Build history of the part. All positions in model axes, mm. A direction names the side the tool comes from. Give positions to 0.01 mm unless a question says otherwise; leave off trailing zeros. Order: outer loops, then holes, each group sorted by start corner. A loop starts at its lowest first (then second) coordinate and runs counter-clockwise, first axis right, second up. Notation, with made-up numbers: M 18.25,-23.5 L 48.25,-23.5 A22 cw 48.25,-6.5 Z; hole C 31.5,34 d11. An arc over 180 degrees is marked long. One line per item, written item: value.
from build123d import *

# Parameters (mm, degrees)
SKETCH1_R                                           = 14
BOSS_EXTRUDE1_DEPTH                                 = 37
SKETCH2_W                                           = 37
SKETCH2_H                                           = 37
BOSS_EXTRUDE2_DEPTH                                 = 6
CUT_EXTRUDE1_DEPTH                                  = 46.315560241
CBORE_FOR_M4_HEX_SOCKET_HEAD_CAP_SCREW1_D           = 4.5
CBORE_FOR_M4_HEX_SOCKET_HEAD_CAP_SCREW1_DEPTH       = 22
CBORE_FOR_M4_HEX_SOCKET_HEAD_CAP_SCREW1_CBORE_D     = 8
CBORE_FOR_M4_HEX_SOCKET_HEAD_CAP_SCREW1_CBORE_DEPTH = 4.4
CBORE_FOR_M4_HEX_SOCKET_HEAD_CAP_SCREW1_TIP         = 1.351936393
SKETCH8_R                                           = 8
CUT_EXTRUDE2_DEPTH                                  = 46.315560241
CHAMFER1_SIZE                                       = 1


with BuildPart() as part:
    # Sketch1 → Boss-Extrude1 (new body)
    with BuildSketch(Plane.XY):
        Circle(SKETCH1_R)
    extrude(amount=BOSS_EXTRUDE1_DEPTH)

    # Sketch2 → Boss-Extrude2 (add)
    with BuildSketch(Plane.XY.offset(37)):
        Rectangle(SKETCH2_W, SKETCH2_H)
    extrude(amount=-BOSS_EXTRUDE2_DEPTH)

    # Sketch4 → Cut-Extrude1 (cut, through all)
    with BuildSketch(Plane.XY.offset(37)):
        Polygon((-18.5, 18.5), (-18.5, 15.441125497), (-15.441125497, 18.5), align=None)
        Polygon((15.441125497, 18.5), (18.5, 18.5), (18.5, 15.441125497), align=None)
        Polygon((18.5, -18.5), (18.5, -15.441125497), (15.441125497, -18.5), align=None)
        Polygon((-15.441125497, -18.5), (-18.5, -18.5), (-18.5, -15.441125497), align=None)
    extrude(amount=-CUT_EXTRUDE1_DEPTH, mode=Mode.SUBTRACT)

    # CBORE for M4 Hex Socket Head Cap Screw1
    with Locations(Plane.XY.offset(37)):
        with Locations((-13.435028843, 13.435028843), (13.435028843, 13.435028843), (13.435028843, -13.435028843), (-13.435028843, -13.435028843)):
            CounterBoreHole(CBORE_FOR_M4_HEX_SOCKET_HEAD_CAP_SCREW1_D / 2, CBORE_FOR_M4_HEX_SOCKET_HEAD_CAP_SCREW1_CBORE_D / 2, CBORE_FOR_M4_HEX_SOCKET_HEAD_CAP_SCREW1_CBORE_DEPTH, depth=CBORE_FOR_M4_HEX_SOCKET_HEAD_CAP_SCREW1_DEPTH)
            with Locations((0, 0, -(CBORE_FOR_M4_HEX_SOCKET_HEAD_CAP_SCREW1_DEPTH + CBORE_FOR_M4_HEX_SOCKET_HEAD_CAP_SCREW1_TIP / 2))):  # 118° drill point
                Cone(0, CBORE_FOR_M4_HEX_SOCKET_HEAD_CAP_SCREW1_D / 2, CBORE_FOR_M4_HEX_SOCKET_HEAD_CAP_SCREW1_TIP, mode=Mode.SUBTRACT)

    # Sketch8 → Cut-Extrude2 (cut, through all)
    with BuildSketch(Plane.XY.offset(37)):
        Circle(SKETCH8_R)
    extrude(amount=-CUT_EXTRUDE2_DEPTH, mode=Mode.SUBTRACT)

    # Chamfer1
    chamfer1_edges = [part.edges().sort_by_distance(p)[0] for p in [
        (-8, 0, 37),
        (-14, 0, 0),
    ]]
    chamfer(chamfer1_edges, length=CHAMFER1_SIZE)


solid = part.part
1) Saw through at A-A, the plane y = 0. Write the cut outline in (x, z).
Check values:
outline: M -18.5,31 L -14,31 L -14,1 L -13,0 L -8,0 L -8,36 L -9,37 L -18.5,37 Z; M 8,0 L 13,0 L 14,1 L 14,31 L 18.5,31 L 18.5,37 L 9,37 L 8,36 Z
2) Mould opens along X. For faces 1 (the face through (6, 6, 0)), 2 (the face through (-16.99, -16.95, 34.04)), 3 (the face through (-9.62, -12.23, 34.83)) say: released by +X, released by -X, zero draft, split by the parting line, or undercut.
Check values:
face 1: zero draft
face 2: released by -X
face 3: undercut
3) Pin check, flat tips, straight feed: pin 1 (9 mm diameter, centred on x = 13.44, y = -13.44, fed in from -Z); pin 2 (12 mm diameter, centred on y = 1.5, z = 17.5, fed in from -X); pin 3 (4 mm diameter, centred on x = 13.44, y = 13.44, fed in from -Z); pin 4 (4 mm diameter, centred on x = -14.5, y = -14, fed in from +Z). Stop position of each tip, or through.
Check values:
pin 1: z = 31
pin 2: x = -14
pin 3: through
pin 4: z = 32.6
4) Drill centre lines: probe 1 along X at (y, z) = (16, 33); probe 2 along Y at (x, z) = (1.5, 27.5); probe 3 along Y at (x, z) = (1, 22.5). Where is each one in solid material? Low to high. Write a range as from..to.
Check values:
probe 1: -17.94..-16.5, -10.37..10.37, 16.5..17.94
probe 2: -13.92..-7.86, 7.86..13.92
probe 3: -13.96..-7.94, 7.94..13.96
5) Saw through at D-D, the plane x = -12. Give the number of separate pieces and of enclosed holes in the cut face, then the cut area to 3 significant figures.
Check values:
separate pieces: 3
enclosed holes: 0
area: 590 mm^2
6) Tool access for faces 4 (the face through (-15.58, -12.76, 31.79)), 5 (the face through (12.932, -5.362, 15.79)), 6 (the face through (15.2, -15.2, 32.6)): list every direction of +Z, -Z, +X, -X, +Y, -Y with a clear straight run to the whole face (end or side of a thin tool).
Check values:
face 4: +Z, -Z
face 5: -Z
face 6: +Z
7) Saw through at C-C, the plane z = 17. Write the cut outline in (x, y).
Check values:
outline: C 0,0 d28; hole C 0,0 d16
